```python
from build123d import *

# Parameters (mm, degrees)
ESQUISSE1_W             = 108.59
ESQUISSE1_H             = 108.59
ESQUISSE1_R             = 1.8
BOSS_EXTRU_1_DEPTH      = 5
ESQUISSE2_W             = 54.295
ESQUISSE2_H             = 7
BOSS_EXTRU_2_DEPTH      = 35
ESQUISSE3_R             = 1
BOSS_EXTRU_3_DEPTH      = 3
ESQUISSE4_W             = 8.59995714
ESQUISSE4_H             = 23.592650329
ENL_V_MAT_EXTRU_1_DEPTH = 5


with BuildPart() as part:
    # Esquisse1 → Boss.-Extru.1 (new body)
    with BuildSketch(Plane(origin=(0, 0, 0), x_dir=(-1, 0, 0), z_dir=(0, 0, 1))):
        with Locations((42.529454852, 77.182817805)):
            Rectangle(ESQUISSE1_W, ESQUISSE1_H)
        with Locations(Location((-1.765545148, 121.477817805, 0), (0, 0, 180))):
            Circle(ESQUISSE1_R, mode=Mode.SUBTRACT)
        with Locations(Location((86.824454852, 121.477817805, 0), (0, 0, 180))):
            Circle(ESQUISSE1_R, mode=Mode.SUBTRACT)
        with Locations(Location((86.824454852, 32.887817805, 0), (0, 0, 180))):
            Circle(ESQUISSE1_R, mode=Mode.SUBTRACT)
        with Locations(Location((-1.765545148, 32.887817805, 0), (0, 0, 180))):
            Circle(ESQUISSE1_R, mode=Mode.SUBTRACT)
        with Locations(Location((42.529454852, 32.887817805, 0), (0, 0, 180))):
            Circle(ESQUISSE1_R, mode=Mode.SUBTRACT)
        with Locations(Location((42.529454852, 121.477817805, 0), (0, 0, 180))):
            Circle(ESQUISSE1_R, mode=Mode.SUBTRACT)
    extrude(amount=BOSS_EXTRU_1_DEPTH)

    # Esquisse2 → Boss.-Extru.2 (add)
    with BuildSketch(Plane.XY.offset(5)):
        with Locations((-15.381954852, -97.182817805)):
            Rectangle(ESQUISSE2_W, ESQUISSE2_H)
        Polygon((-42.529454852, -60.682817805), (-42.529454852, -53.682817805), (-49.529454852, -53.682817805), (-49.529454852, -100.682817805), (-42.529454852, -100.682817805), (-42.529454852, -93.682817805), (-42.529454852, -77.182817805), align=None)
        with Locations((-15.381954852, -57.182817805)):
            Rectangle(ESQUISSE2_W, ESQUISSE2_H)
    extrude(amount=BOSS_EXTRU_2_DEPTH)

    # Esquisse3 → Boss.-Extru.3 (add)
    with BuildSketch(Plane.XY.offset(40)):
        Polygon((11.765545148, -53.682817805), (-49.529454852, -53.682817805), (-49.529454852, -100.682817805), (11.765545148, -100.682817805), (11.765545148, -88.982817805), (-42.529454852, -88.982817805), (-42.529454852, -65.390167476), (11.765545148, -65.390167476), align=None)
        with Locations((-24.229454852, -90.682817805)):
            Circle(ESQUISSE3_R, mode=Mode.SUBTRACT)
        with BuildLine():
            ThreePointArc((-15.229454852, -90.682817805), (-16.229454852, -91.682817805), (-17.229454852, -90.682817805))
            ThreePointArc((-17.229454852, -90.682817805), (-16.229454852, -89.682817805), (-15.229454852, -90.682817805))
        make_face(mode=Mode.SUBTRACT)
        with BuildLine():
            ThreePointArc((-7.229454852, -90.682817805), (-8.229454852, -91.682817805), (-9.229454852, -90.682817805))
            ThreePointArc((-9.229454852, -90.682817805), (-8.229454852, -89.682817805), (-7.229454852, -90.682817805))
        make_face(mode=Mode.SUBTRACT)
        with Locations((-0.229454852, -90.682817805)):
            Circle(ESQUISSE3_R, mode=Mode.SUBTRACT)
        with Locations((-24.229454852, -63.682817805)):
            Circle(ESQUISSE3_R, mode=Mode.SUBTRACT)
        with BuildLine():
            ThreePointArc((-15.229454852, -63.682817805), (-16.229454852, -64.682817805), (-17.229454852, -63.682817805))
            ThreePointArc((-17.229454852, -63.682817805), (-16.229454852, -62.682817805), (-15.229454852, -63.682817805))
        make_face(mode=Mode.SUBTRACT)
        with BuildLine():
            ThreePointArc((-7.229454852, -63.682817805), (-8.229454852, -64.682817805), (-9.229454852, -63.682817805))
            ThreePointArc((-9.229454852, -63.682817805), (-8.229454852, -62.682817805), (-7.229454852, -63.682817805))
        make_face(mode=Mode.SUBTRACT)
        with Locations((-0.229454852, -63.682817805)):
            Circle(ESQUISSE3_R, mode=Mode.SUBTRACT)
    extrude(amount=BOSS_EXTRU_3_DEPTH)

    # Esquisse4 → Enl_v. mat.-Extru.1 (cut)
    with BuildSketch(Plane.XY.offset(5)):
        with Locations((-18.074099951, -77.186492641)):
            Rectangle(ESQUISSE4_W, ESQUISSE4_H)
    extrude(amount=-ENL_V_MAT_EXTRU_1_DEPTH, mode=Mode.SUBTRACT)

    # Esquisse5 → Lissage3 section 0
    with BuildSketch(Plane.ZY.offset(49.529454852)):
        with BuildLine():
            Line((43, -100.682817805), (38, -100.682817805))
            Line((38, -100.682817805), (38, -53.682817805))
            Line((38, -53.682817805), (43, -53.682817805))
            Line((43, -53.682817805), (43, -100.682817805))
        make_face()
    # Esquisse6 → Lissage3 section 1
    with BuildSketch(Plane.XY.offset(5)):
        with BuildLine():
            Line((-74.529454852, -115.182817805), (-74.529454852, -39.182817805))
            Line((-74.529454852, -39.182817805), (-70.204298905, -41.691408254))
            Line((-70.204298905, -41.691408254), (-70.204298905, -112.674227356))
            Line((-70.204298905, -112.674227356), (-74.529454852, -115.182817805))
        make_face()
    loft()


solid = part.part
```
Input: part model. Units: mm. Frame: model coordinates. A direction names the side the tool comes from. Coordinates: 2 decimals unless noted, no trailing zeros. Write each loop counter-clockwise with the first axis right and the second up, starting at its lowest first coordinate (ties: lowest second). Pieces come first, ordered by that corner, then holes. Notation, with made-up numbers: (70, 4) - (80, 4) arc R12 cw to (80, 25) - close; hole circle Ø6 at (-26, 78.5). An arc over 180 degrees is marked (long way). Put each result on its own line as item: value. Start each with the question number.
1) Contact query for flat-ended pins moving along their axis: pin 1 (12 mm diameter, centred on x = -82.5, y = -112, fed in from +Z); pin 2 (3 mm diameter, centred on x = -42.53, y = -121.48, fed in from -Z) (1 decimal); pin 3 (6 mm diameter, centred on x = -1, z = 21, fed in from -Y); pin 4 (10 mm diameter, centred on x = -21.5, z = 24, fed in from +Y). Output: stop coordinate, or through.
2) Cut plane B-B (z = 3). Return the cut outline in (x, y), plus the area to 3 significant figures.
3) Reachability of faces 5 (the face through (-15, -88.983, 41)), 6 (the face through (-18, -65.39, 3)), 7 (the face through (-16, -62, 40)) from +Z, -Z, +X, -X, +Y, -Y: full face, straight path, thin tool, end or side. Return the list, or none.
4) Ray query, L1, parallel to Y at x = -13.5, z = 14; L2, parallel to X at y = -78.5, z = 4.5; L3, parallel to Z at x = -44.5, y = -31. Return the intervals inside material, ascending.
5) Cut plane A-A (y = -69.5). State how many separate pieces and enclosed holes the cut face has, plus the area to 3 significant figures.
6) Cut plane C-C (x = -81). Return the cut outline in (y, z), plus the area to 3 significant figures.
7) Mould query, pull axis Y, two halves, no side actions, for faces 1 (the face through (-85.108, -120.937, 2.465)), 2 (the face through (-16, -60.683, 22)), 3 (the face through (-19, -100.683, 24)), 4 (the face through (-96.824, -76, 2)). Classes: pulls with the +Y half, pulls with the -Y half, needs draft (parallel to the pull), parting line crosses it, or undercut.
Resolved:
1. pin 1: stops at z = 5
1. pin 2: passes through
1. pin 3: stops at y = -100.68
1. pin 4: stops at y = -53.68
2. outline: (-96.82, -131.48) - (11.77, -131.48) - (11.77, -22.89) - (-96.82, -22.89) - close; hole circle Ø3.6 at (-86.82, -121.48); hole circle Ø3.6 at (-86.82, -32.89); hole circle Ø3.6 at (-42.53, -121.48); hole circle Ø3.6 at (-42.53, -32.89); hole (-22.37, -88.98) - (-13.77, -88.98) - (-13.77, -65.39) - (-22.37, -65.39) - close; hole circle Ø3.6 at (1.77, -121.48); hole circle Ø3.6 at (1.77, -32.89)
2. area: 11,500 mm2
3. face 5: +Z, +X
3. face 6: +Z, -Z
3. face 7: +X
4. L1: y = -100.68 to -93.68, -60.68 to -53.68
4. L2: x = -96.82 to -22.37, -13.77 to 11.77
4. L3: z = 0 to 5
5. separate pieces: 2
5. enclosed holes: 1
5. area: 900 mm2
6. outline: (-131.48, 0) - (-22.89, 0) - (-22.89, 5) - (-131.48, 5) - close
6. area: 543 mm2
7. face 1: undercut
7. face 2: undercut
7. face 3: pulls with the -Y half
7. face 4: needs draft
